Could you check a few things on this drawing? It's one solid part, dimensions in mm from its lowest x, y, z. Give positions to 0.01 mm unless a question says otherwise; leave off trailing zeros. Loops run counter-clockwise (first coordinate to the right, second up) from the corner with the lowest first, then second, coordinate; pieces in that order, holes last. Notation, with made-up numbers: (72, 55.25) - (121, 55.25) arc R18 ccw to (121, 77.25) - close; hole circle Ø11 at (58.25, 63.25). An arc over 180 degrees is marked (long way). Use a Markdown table: item, result.
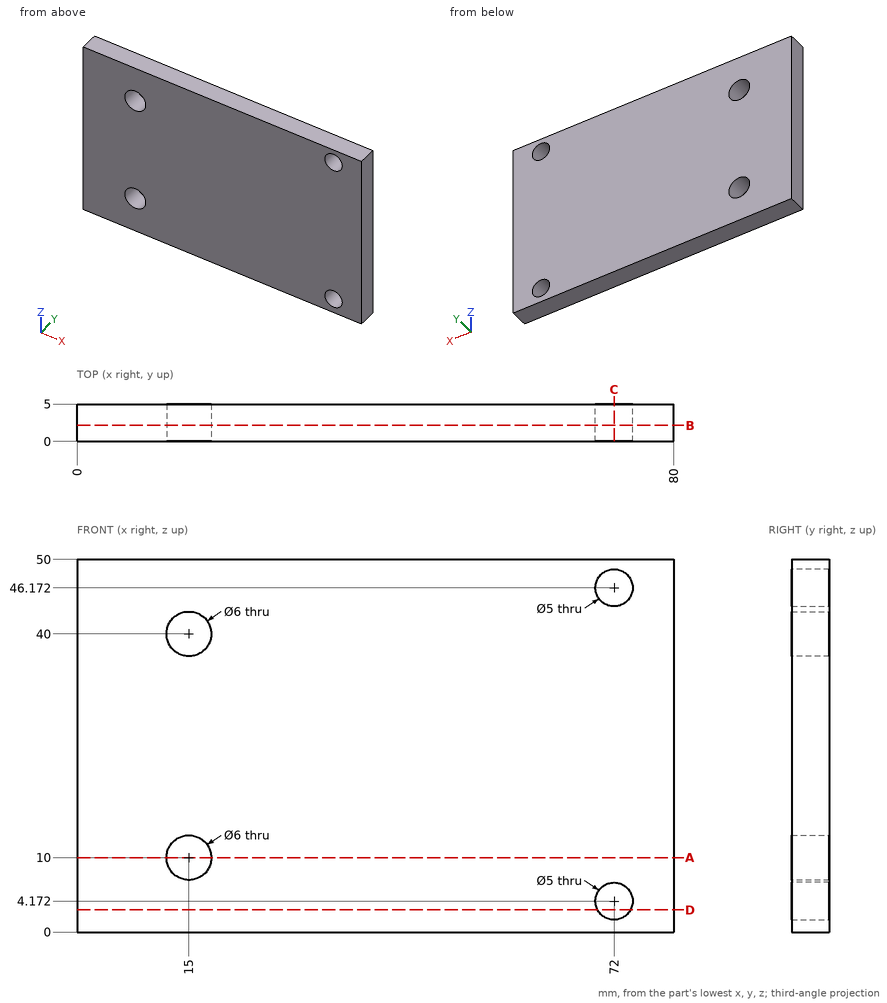
(1) Suppose I cut it at B-B on y = 2.15. Write out the boundary of the cut face in (x, z).
A:
| item | result |
|---|---|
| outline | (0, 0) - (80, 0) - (80, 50) - (0, 50) - close; hole circle Ø6 at (15, 10); hole circle Ø6 at (15, 40); hole circle Ø5 at (72, 4.17); hole circle Ø5 at (72, 46.17) |
(2) Suppose I cut it at C-C on x = 72. Write out the boundary of the cut face in (y, z).
A:
| item | result |
|---|---|
| outline | (0, 0) - (5, 0) - (5, 1.67) - (0, 1.67) - close; (0, 6.67) - (5, 6.67) - (5, 43.67) - (0, 43.67) - close; (0, 48.67) - (5, 48.67) - (5, 50) - (0, 50) - close |
(3) Suppose I cut it at D-D on z = 3. Write out the boundary of the cut face in (x, y).
A:
| item | result |
|---|---|
| outline | (0, 0) - (69.79, 0) - (69.79, 5) - (0, 5) - close; (74.21, 0) - (80, 0) - (80, 5) - (74.21, 5) - close |
(4) Will this pin go through, and if not, where does the flat tip stop? pin 1 (12 mm diameter, centred on x = 30.5, z = 41, fed in from -Y).
A:
| item | result |
|---|---|
| pin 1 | y = 0 |
(5) Suppose I cut it at A-A on z = 10. Write out the boundary of the cut face in (x, y), plus the area to 3 significant figures.
A:
| item | result |
|---|---|
| outline | (0, 0) - (12, 0) - (12, 5) - (0, 5) - close; (18, 0) - (80, 0) - (80, 5) - (18, 5) - close |
| area | 370 mm2 |
(6) If I drill on line 1 (X direction, y = 2.1, z = 10); line 2 (X direction, y = 0.8, z = 42.5), over which ranges is the centre line in solid material (lowest first)?
A:
| item | result |
|---|---|
| line 1 | 0 to 12, 18 to 80 |
| line 2 | 0 to 13.34, 16.66 to 80 |
